from build123d import *

# Parameters (mm, degrees)
SKETCH1_W           = 685
SKETCH1_H           = 250
BASE_FLANGE1_DEPTH  = 8
SKETCH6_W           = 60
SKETCH6_H           = 8
SKETCH6_W_2         = 70
EXTRUDE1_DEPTH      = 8
SKETCH7_W           = 250
SKETCH7_H           = 73.5
BASE_FLANGE2_DEPTH  = 8
SKETCH12_W          = 30.5
SKETCH12_H          = 8.5
EXTRUDE2_DEPTH      = 699.681794525
SKETCH14_W          = 250
SKETCH14_H          = 8
BASE_FLANGE3_DEPTH  = 50.5
SKETCH19_W          = 60
SKETCH19_H          = 8
SKETCH19_W_2        = 70
EXTRUDE3_DEPTH      = 8
BREAK_CORNER1_START = 41.5
BREAK_CORNER1_DEPTH = 8
EXTRUDE4_DEPTH      = 8
BASE_FLANGE4_DEPTH  = 8
SKETCH38_W          = 8.5
SKETCH38_H          = 20.5
EXTRUDE5_DEPTH      = 10
SKETCH39_W          = 20.5
SKETCH39_H          = 8.5
EXTRUDE6_DEPTH      = 10


# Read off the part's stored shape, not the designer's step: Break-Corner1
# Sheet-metal steps are written as plain solids
with BuildPart() as part:
    # Sketch1 → Base-Flange1 (new body)
    with BuildSketch(Plane(origin=(0, 0, 0), x_dir=(1, 0, 0), z_dir=(0, 1, 0))):
        Rectangle(SKETCH1_W, SKETCH1_H)
    extrude(amount=-BASE_FLANGE1_DEPTH)

    # Sketch6 → Extrude1 (cut)
    with BuildSketch(Plane(origin=(342.5, 0, 0), x_dir=(0, 0, -1), z_dir=(1, 0, 0))):
        with Locations((-95, -4)):
            Rectangle(SKETCH6_W, SKETCH6_H)
        with Locations((95, -4)):
            Rectangle(SKETCH6_W, SKETCH6_H)
        with Locations((0, -4)):
            Rectangle(SKETCH6_W_2, SKETCH6_H)
    extrude1 = extrude(amount=-EXTRUDE1_DEPTH, mode=Mode.SUBTRACT)

    # Mirror1: Extrude1 across plane
    add(extrude1.mirror(Plane(origin=(0, 0, 0), x_dir=(0, 0, 1), z_dir=(1, 0, 0))), mode=Mode.SUBTRACT)

    # Sketch39 → Extrude6 (cut)
    with BuildSketch(Plane.XZ.offset(8)):
        with Locations((289.5, 0)):
            Rectangle(SKETCH39_W, SKETCH39_H)
        with Locations((229.5, 0)):
            Rectangle(SKETCH39_W, SKETCH39_H)
        with Locations((-289.5, 0)):
            Rectangle(SKETCH39_W, SKETCH39_H)
        with Locations((-229.5, 0)):
            Rectangle(SKETCH39_W, SKETCH39_H)
    extrude(amount=-EXTRUDE6_DEPTH, mode=Mode.SUBTRACT)


with BuildPart() as body_2:
    # Sketch7 → Base-Flange2 (new body)
    with BuildSketch(Plane(origin=(334.5, 0, 0), x_dir=(0, 0, -1), z_dir=(1, 0, 0))):
        with Locations((0, 20.75)):
            Rectangle(SKETCH7_W, SKETCH7_H)
    extrude(amount=BASE_FLANGE2_DEPTH)

    # Sketch12 → Extrude2 (cut, through all)
    with BuildSketch(Plane(origin=(342.5, 0, 0), x_dir=(0, 0, -1), z_dir=(1, 0, 0))):
        with Locations((-50, -4)):
            Rectangle(SKETCH12_W, SKETCH12_H)
        with Locations((50, -4)):
            Rectangle(SKETCH12_W, SKETCH12_H)
        with Locations((50, 45.5)):
            Rectangle(SKETCH12_W, SKETCH12_H)
        with Locations((-50, 45.5)):
            Rectangle(SKETCH12_W, SKETCH12_H)
    extrude(amount=-EXTRUDE2_DEPTH, mode=Mode.SUBTRACT)

    # Sketch38 → Extrude5 (cut)
    with BuildSketch(Plane(origin=(342.5, 0, 0), x_dir=(0, 0, -1), z_dir=(1, 0, 0))):
        with Locations((0, 27.5)):
            Rectangle(SKETCH38_W, SKETCH38_H)
    extrude(amount=-EXTRUDE5_DEPTH, mode=Mode.SUBTRACT)


with BuildPart() as body_3:
    # Sketch14 → Base-Flange3 (new body)
    with BuildSketch(Plane.ZY.offset(-334.5)):
        with Locations((0, 45.5)):
            Rectangle(SKETCH14_W, SKETCH14_H)
    extrude(amount=-BASE_FLANGE3_DEPTH)

    # Sketch19 → Extrude3 (cut)
    with BuildSketch(Plane(origin=(342.5, 0, 0), x_dir=(0, 0, -1), z_dir=(1, 0, 0))):
        with Locations((95, 45.5)):
            Rectangle(SKETCH19_W, SKETCH19_H)
        with Locations((0, 45.5)):
            Rectangle(SKETCH19_W_2, SKETCH19_H)
        with Locations((-95, 45.5)):
            Rectangle(SKETCH19_W, SKETCH19_H)
    extrude(amount=-EXTRUDE3_DEPTH, mode=Mode.SUBTRACT)

    # Break-Corner1 outline → Break-Corner1 (cut)
    with BuildSketch(Plane(origin=(0, 0, 0), x_dir=(1, 0, 0), z_dir=(0, 1, 0)).offset(BREAK_CORNER1_START)):
        Polygon((385, -125), (385, -110), (370, -125), align=None)
        Polygon((370, 125), (385, 110), (385, 125), align=None)
    extrude(amount=BREAK_CORNER1_DEPTH, mode=Mode.SUBTRACT)

    # Sketch20 → Extrude4 (cut)
    with BuildSketch(Plane(origin=(0, 49.5, 0), x_dir=(1, 0, 0), z_dir=(0, 1, 0))):
        with BuildLine():
            Line((367, 75), (367, 55))
            ThreePointArc((367, 55), (362.5, 50.5), (358, 55))
            Line((358, 55), (358, 75))
            ThreePointArc((358, 75), (362.5, 79.5), (367, 75))
        make_face()
        with BuildLine():
            Line((367, -75), (367, -55))
            ThreePointArc((367, -55), (362.5, -50.5), (358, -55))
            Line((358, -55), (358, -75))
            ThreePointArc((358, -75), (362.5, -79.5), (367, -75))
        make_face()
    extrude(amount=-EXTRUDE4_DEPTH, mode=Mode.SUBTRACT)


with BuildPart() as body_4:
    # Mirror4: mirrored copy
    add(body_3.part.mirror(Plane(origin=(0, 0, 0), x_dir=(0, 0, 1), z_dir=(1, 0, 0))))


with BuildPart() as body_5:
    # Sketch29 → Base-Flange4 (new body)
    with BuildSketch(Plane.XY.offset(4)):
        Polygon((219.5, 0), (219.5, -8), (239.5, -8), (239.5, 0), (279.5, 0), (279.5, -8), (299.5, -8), (299.5, 0), (334.5, 0), (334.5, 17.5), (342.5, 17.5), (342.5, 37.5), (334.5, 37.5), (334.5, 57.5), (194.5, 10), (194.5, 0), align=None)
    extrude(amount=-BASE_FLANGE4_DEPTH)


with BuildPart() as body_6:
    # Mirror5: mirrored copy
    add(body_5.part.mirror(Plane(origin=(0, 0, 0), x_dir=(0, 0, 1), z_dir=(1, 0, 0))))


with BuildPart() as body_7:
    # Mirror3: mirrored copy
    add(body_2.part.mirror(Plane(origin=(0, 0, 0), x_dir=(0, 0, 1), z_dir=(1, 0, 0))))


solid = body_6.part
Verification items for the finished model (mm, model axes). A direction names the side the tool comes from. Coordinates: 2 decimals unless noted, no trailing zeros. Write each loop counter-clockwise with the first axis right and the second up, starting at its lowest first coordinate (ties: lowest second). Pieces come first, ordered by that corner, then holes. Notation, with made-up numbers: (42.25, 52) -> (69.25, 52) arc R26 cw to (69.25, 79) -> close; hole circle Ø2 at (24.5, 89.5). An arc over 180 degrees is marked (long way). One line per item, written item: value. Start each with the question number.
Q1. Cross-section at C-C on x = -314. Enter the section's corners in (y, z), and give its area (3 significant figures).
Q2. Access from +Z, -Z, +X, -X, +Y, -Y to the whole of each face (thin tool, end or side, straight path). Record for faces 1 (the flat face through (-219.5, -4, 0)), 2 (the flat face through (-339, 37.5, 0)), 3 (the flat face through (-299.5, -4, 0)), 4 (the flat face through (-239.5, -4, 0)).
Q3. Cross-section at A-A on z = -1.75. Enter the section's corners in (x, y).
Q4. Mould release check, pull along X, two halves, no side actions. Record for faces 5 (the flat face through (-289, -8, 0)), 6 (the flat face through (-279.5, -4, 0)), 7 (the flat face through (-265.48, 34.082, 0.056)), 8 (the flat face through (-259, 0, 0)): pulls with the +X half, pulls with the -X half, needs draft (parallel to the pull), parting line crosses it, or undercut.
Q5. Thickness scan on L1, parallel to X at y = -4.5, z = -1; L2, parallel to X at y = 9, z = -2.25; L3, parallel to Y at x = -269, z = 0.25. Record the ranges inside material, lowest first. Write a range as from..to.
Q6. Go/stop test with flat-tipped pins: P1, Ø4, axis at x = -337, z = 2, coming from the +Y side; P2, Ø4, axis at y = 49, z = 0, coming from the -X side; P3, Ø2.5, axis at x = -210, z = -0.5, coming from the -Y side. Record where each tip stops, or that it passes through.
Q7. Cross-section at B-B on y = 7.5. Enter the section's corners in (x, z).
Checked values:
1. outline: (0, -4) -> (50.54, -4) -> (50.54, 4) -> (0, 4) -> close
1. area: 404 mm²
2. face 1: +Z, -Z, +X, -Y
2. face 2: +Z, -Z, -X, +Y
2. face 3: +Z, -Z, -X, -Y
2. face 4: +Z, -Z, -Y
3. outline: (-342.5, 17.5) -> (-334.5, 17.5) -> (-334.5, 0) -> (-299.5, 0) -> (-299.5, -8) -> (-279.5, -8) -> (-279.5, 0) -> (-239.5, 0) -> (-239.5, -8) -> (-219.5, -8) -> (-219.5, 0) -> (-194.5, 0) -> (-194.5, 10) -> (-334.5, 57.5) -> (-334.5, 37.5) -> (-342.5, 37.5) -> close
4. face 5: needs draft
4. face 6: undercut
4. face 7: pulls with the +X half
4. face 8: undercut
5. L1: x = -299.5..-279.5, -239.5..-219.5
5. L2: x = -334.5..-194.5
5. L3: y = 0..35.28
6. P1: stops at y = 37.5
6. P2: stops at x = -334.5
6. P3: stops at y = 0
7. outline: (-334.5, -4) -> (-194.5, -4) -> (-194.5, 4) -> (-334.5, 4) -> close
